from build123d import *

# Parameters (mm, degrees)
SKETCH1_W           = 88.9
SKETCH1_H           = 25.4
BOSS_EXTRUDE1_DEPTH = 14.999999972
SKETCH2_W           = 14.499999956
SKETCH2_H           = 6.99999997
CUT_EXTRUDE1_DEPTH  = 25.4
SKETCH3_R           = 1.27
CUT_EXTRUDE3_DEPTH  = 25.4


with BuildPart() as part:
    # Sketch1 → Boss-Extrude1 (new body)
    with BuildSketch(Plane(origin=(0, 0, 0), x_dir=(1, 0, 0), z_dir=(0, 1, 0))):
        Rectangle(SKETCH1_W, SKETCH1_H)
    extrude(amount=BOSS_EXTRUDE1_DEPTH)

    # Sketch2 → Cut-Extrude1 (cut)
    with BuildSketch(Plane(origin=(0, 14.999999972, 0), x_dir=(1, 0, 0), z_dir=(0, 1, 0))):
        Rectangle(SKETCH2_W, SKETCH2_H)
        with Locations((-28.430000036, 0)):
            Rectangle(SKETCH2_W, SKETCH2_H)
        with Locations((28.430000036, 0)):
            Rectangle(SKETCH2_W, SKETCH2_H)
    extrude(amount=-CUT_EXTRUDE1_DEPTH, mode=Mode.SUBTRACT)

    # Sketch3 → Cut-Extrude3 (cut)
    with BuildSketch(Plane(origin=(0, 14.999999972, 0), x_dir=(1, 0, 0), z_dir=(0, 1, 0))):
        with Locations((-40.45, 8.7)):
            Circle(SKETCH3_R)
        with Locations((40.45, 8.7)):
            Circle(SKETCH3_R)
        with Locations((-40.45, -8.7)):
            Circle(SKETCH3_R)
        with Locations((40.45, -8.7)):
            Circle(SKETCH3_R)
    extrude(amount=-CUT_EXTRUDE3_DEPTH, mode=Mode.SUBTRACT)


solid = part.part
Source: CAD feature listing. Evaluate the final solid. Frame: model axes, mm. A direction names the side the tool comes from. Round coordinates to 2 decimals unless told otherwise and drop trailing zeros. Loops run counter-clockwise (first coordinate to the right, second up) from the corner with the lowest first, then second, coordinate; pieces in that order, holes last.
Q1. Access query for faces 5 (the face through (-1, 15, 5)), 6 (the face through (-35.68, 8, 0)). Directions: +Z, -Z, +X, -X, +Y, -Y. A direction counts if a zero-diameter tool reaches every point of the face in a straight line with its end or side. Return the directions, or none.
Q2. Mould query, pull axis Z, two halves, no side actions, for faces 1 (the face through (7.25, 8, 0)), 2 (the face through (-1, 7, -12.7)), 3 (the face through (-44.45, 7, 0)), 4 (the face through (-1, 7, 12.7)). Classes: pulls with the +Z half, pulls with the -Z half, needs draft (parallel to the pull), parting line crosses it, or undercut.
Q3. Section B-B, the plane z = -2.75. Return loops of the section in (x, y), plus the area to 3 significant figures.
Q4. Section A-A, the plane x = -34.5. Return loops of the section in (y, z).
Q5. Section D-D, the plane z = 8.7. Return loops of the section in (x, y), plus the area to 3 significant figures.
Q6. Ray query, line 1 (X direction, y = 3, z = 0.5); line 2 (Z direction, x = 40.45, y = 8.5); line 3 (X direction, y = 7, z = -8.7). Return the intervals inside material, ascending.
Q7. Section C-C, the plane y = 7.5. Return loops of the section in (x, z).
Solutions:
1. face 5: +Z, -Z, +X, -X, +Y
1. face 6: +Y, -Y
2. face 1: undercut
2. face 2: pulls with the -Z half
2. face 3: needs draft
2. face 4: pulls with the +Z half
3. outline: (-44.45, 0) - (-35.68, 0) - (-35.68, 15) - (-44.45, 15) - close; (-21.18, 0) - (-7.25, 0) - (-7.25, 15) - (-21.18, 15) - close; (7.25, 0) - (21.18, 0) - (21.18, 15) - (7.25, 15) - close; (35.68, 0) - (44.45, 0) - (44.45, 15) - (35.68, 15) - close
3. area: 681 mm2
4. outline: (0, -12.7) - (15, -12.7) - (15, -3.5) - (0, -3.5) - close; (0, 3.5) - (15, 3.5) - (15, 12.7) - (0, 12.7) - close
5. outline: (-44.45, 0) - (-41.72, 0) - (-41.72, 15) - (-44.45, 15) - close; (-39.18, 0) - (39.18, 0) - (39.18, 15) - (-39.18, 15) - close; (41.72, 0) - (44.45, 0) - (44.45, 15) - (41.72, 15) - close
5. area: 1,260 mm2
6. line 1: x = -44.45 to -35.68, -21.18 to -7.25, 7.25 to 21.18, 35.68 to 44.45
6. line 2: z = -12.7 to -9.97, -7.43 to 7.43, 9.97 to 12.7
6. line 3: x = -44.45 to -41.72, -39.18 to 39.18, 41.72 to 44.45
7. outline: (-44.45, -12.7) - (44.45, -12.7) - (44.45, 12.7) - (-44.45, 12.7) - close; hole circle Ø2.54 at (-40.45, -8.7); hole circle Ø2.54 at (-40.45, 8.7); hole (-35.68, -3.5) - (-21.18, -3.5) - (-21.18, 3.5) - (-35.68, 3.5) - close; hole (-7.25, -3.5) - (7.25, -3.5) - (7.25, 3.5) - (-7.25, 3.5) - close; hole (21.18, -3.5) - (35.68, -3.5) - (35.68, 3.5) - (21.18, 3.5) - close; hole circle Ø2.54 at (40.45, -8.7); hole circle Ø2.54 at (40.45, 8.7)
